```python
from build123d import *

# Parameters (mm, degrees)
ESQUISSE1_R        = 1.75
BOSS_EXTRU_1_DEPTH = 3
CONG_1_R           = 1.75


with BuildPart() as part:
    # Esquisse1 → Boss.-Extru.1 (new body)
    with BuildSketch(Plane.XY):
        Polygon((-15, -20), (15, -20), (15, 0), (7, 0), (7, 20), (-15, 20), align=None)
        with Locations((12.5, -15)):
            Circle(ESQUISSE1_R, mode=Mode.SUBTRACT)
        with Locations((-12.5, -15)):
            Circle(ESQUISSE1_R, mode=Mode.SUBTRACT)
        with Locations((-12.5, 15)):
            Circle(ESQUISSE1_R, mode=Mode.SUBTRACT)
        with BuildLine():
            ThreePointArc((2.5, 16.5), (3.5, 17.5), (2.5, 18.5))
            Line((2.5, 18.5), (-2.5, 18.5))
            ThreePointArc((-2.5, 18.5), (-3.5, 17.5), (-2.5, 16.5))
            Line((-2.5, 16.5), (2.5, 16.5))
        make_face(mode=Mode.SUBTRACT)
        with BuildLine():
            ThreePointArc((2.5, -13.5), (3.5, -12.5), (2.5, -11.5))
            Line((2.5, -11.5), (-2.5, -11.5))
            ThreePointArc((-2.5, -11.5), (-3.5, -12.5), (-2.5, -13.5))
            Line((-2.5, -13.5), (2.5, -13.5))
        make_face(mode=Mode.SUBTRACT)
        with BuildLine():
            Line((-2.5, -16.5), (2.5, -16.5))
            ThreePointArc((2.5, -16.5), (3.5, -17.5), (2.5, -18.5))
            Line((2.5, -18.5), (-2.5, -18.5))
            ThreePointArc((-2.5, -18.5), (-3.5, -17.5), (-2.5, -16.5))
        make_face(mode=Mode.SUBTRACT)
        with BuildLine():
            Line((-2.5, 13.5), (2.5, 13.5))
            ThreePointArc((2.5, 13.5), (3.5, 12.5), (2.5, 11.5))
            Line((2.5, 11.5), (-2.5, 11.5))
            ThreePointArc((-2.5, 11.5), (-3.5, 12.5), (-2.5, 13.5))
        make_face(mode=Mode.SUBTRACT)
    extrude(amount=BOSS_EXTRU_1_DEPTH)

    # Congé1
    cong_1_edges = [part.edges().sort_by_distance(p)[0] for p in [
        (-15, -20, 1.5),
        (-15, 20, 1.5),
        (7, 20, 1.5),
        (7, 0, 1.5),
        (15, 0, 1.5),
        (15, -20, 1.5),
    ]]
    fillet(cong_1_edges, radius=CONG_1_R)


solid = part.part
```
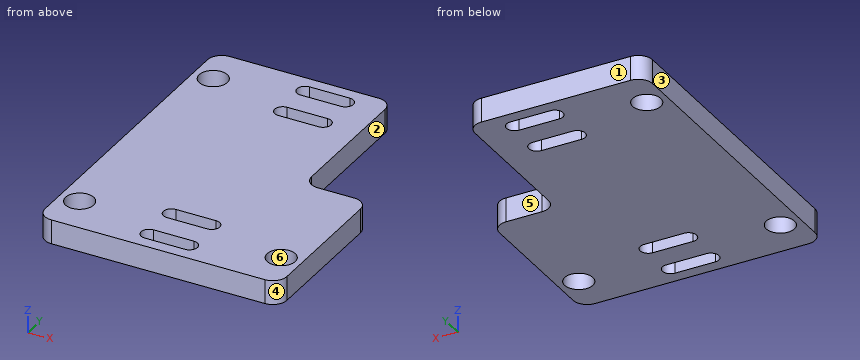
The listing builds one solid part. Answer for the finished solid, in the listing's coordinates (mm). Face numbers are marked on the shaded views. A direction names the side the tool comes from. Coordinates: 2 decimals unless noted, no trailing zeros. Loops run counter-clockwise (first coordinate to the right, second up) from the corner with the lowest first, then second, coordinate; pieces in that order, holes last. Notation, with made-up numbers: M 3,44.25 L 42,44.25 A26 ccw 42,60.25 Z; hole C 46.5,-0.75 d11. An arc over 180 degrees is marked long. Answer as a JSON object with one key per item and string values. Group by question number.
Item 1: Determine the mould class of the marked faces 3, 4, 5 and 6 for opening direction Y: +Y half, -Y half, draft (parallel to the pull), parting line (faces both ways), or undercut.
Item 2: Consider L1, parallel to Y at x = -12.5, z = 0.9; L2, parallel to Y at x = -0.25, z = 1.5; L3, parallel to Y at x = -13.5, z = 1.4. Determine where each line is inside the solid, lowest interval first.
Item 3: This flat-tipped pin is pushed along its axis until it touches: P1, Ø0.9, axis at y = 10, z = 2, coming from the +X side. Where does it stop, or does it pass through?
Item 4: Section D-D (x = 12.5) is taken. Write down the section's boundary in (y, z).
Item 5: Section A-A (x = -12.5) is taken. Write down the section's boundary in (y, z).
Item 6: Section B-B (y = -12.5) is taken. Write down the section's boundary in (x, z), and give its area (3 significant figures).
Item 7: Which of the six approach directions +Z, -Z, +X, -X, +Y, -Y give full straight-line access (tool end or side, diameter ignored) to the marked faces 1 and 2?
Item 8: Section C-C (z = 1.7) is taken. Give the number of separate pieces and of enclosed holes in the cut face, and give its area (3 significant figures).
Solved:
{
 "1": {"face 3": "draft", "face 4": "-Y half", "face 5": "+Y half", "face 6": "undercut"},
 "2": {"L1": "y = -20 to -16.75, -13.25 to 13.25, 16.75 to 20", "L2": "y = -20 to -18.5, -16.5 to -13.5, -11.5 to 11.5, 13.5 to 16.5, 18.5 to 20", "L3": "y = -19.98 to -16.44, -13.56 to 13.56, 16.44 to 19.98"},
 "3": {"P1": "stops at x = 7"},
 "4": {"outline": "M -20,0 L -16.75,0 L -16.75,3 L -20,3 Z; M -13.25,0 L 0,0 L 0,3 L -13.25,3 Z"},
 "5": {"outline": "M -20,0 L -16.75,0 L -16.75,3 L -20,3 Z; M -13.25,0 L 13.25,0 L 13.25,3 L -13.25,3 Z; M 16.75,0 L 20,0 L 20,3 L 16.75,3 Z"},
 "6": {"outline": "M -15,0 L -3.5,0 L -3.5,3 L -15,3 Z; M 3.5,0 L 15,0 L 15,3 L 3.5,3 Z", "area": "69.0 mm2"},
 "7": {"face 1": "+Z, -Z, +X, -X, +Y", "face 2": "+Z, -Z, +X, +Y"},
 "8": {"separate pieces": "1", "enclosed holes": "7", "area": "956 mm2"}
}
